Here's how the part is built. I have some questions about the finished solid (model axes, mm). Coordinates: 2 decimals unless noted, no trailing zeros. Loops run counter-clockwise (first coordinate to the right, second up) from the corner with the lowest first, then second, coordinate; pieces in that order, holes last. Notation, with made-up numbers: M 40.25,32 L 99.25,32 A32 cw 99.25,71 Z; hole C 43.25,60 d10. An arc over 180 degrees is marked long. Use one line per item in the form item = value. Start each with the question number.
(1) Imagine slicing it at D-D, the plane z = 3.35. Please give me the cut outline in (x, y), and give its area (3 significant figures).
(2) Imagine slicing it at C-C, the plane y = -6. Please give me the cut outline in (x, z), and give its area (3 significant figures).
(3) Please list where these lines run through material, in increasing order: L1, parallel to Y at x = 0, z = 3.55; L2, parallel to X at y = 6, z = 2.3; L3, parallel to Y at x = 11.5, z = 0.3.
(4) Will these pins go through, and if not, where does the flat tip stop? P1, Ø2.5, axis at x = 0, y = -12, coming from the +Z side; P2, Ø3, axis at y = 6, z = 2.5, coming from the -X side.
(5) Imagine slicing it at B-B, the plane y = 0. Please give me the cut outline in (x, z).
(6) Thinking about a two-plate mould opening in Y: for faces 1 (the flat face through (8, 0, 5)), 2 (the cylindrical face through (11.701, -4.294, 2.465)), 3 (the cylindrical face through (-4.01, 18.06, 2.46)), which applies, +Y half, -Y half, draft (parallel to the pull), parting line (faces both ways), or undercut?
(7) Imagine slicing it at A-A, the plane x = 0. Please give me the cut outline in (y, z), and give its area (3 significant figures).
Autodesk Inventor part; units mm, degrees
ref_plane "YZ Plane" through (0, 0, 0) normal (1, 0, 0) x (0, 1, 0)
ref_plane "XZ Plane" through (0, 0, 0) normal (0, 1, 0) x (-1, 0, 0)
ref_plane "XY Plane" through (0, 0, 0) normal (0, 0, 1) x (1, 0, 0)
sketch "スケッチ1" plane through (0, 0, 0) normal (0, 0, 1) x (1, 0, 0)
  circle A0 centre (0, 0) radius 18.5
  dimension "d0" = 37
extrude "押し出し1" add sketch "スケッチ1" along normal blind 5
sketch "スケッチ2" plane through (0, 0, 5) normal (0, 0, 1) x (1, 0, 0)
  circle A0 centre (0, 0) radius 12
  point P0 (0, 12)
  point P1 (-10.3923, 6)
  point P2 (-10.3923, -6)
  point P3 (0, -12)
  point P4 (10.3923, -6)
  point P5 (10.3923, 6)
  dimension "d3" = 24
  dimension "d6" = 360
hole "穴1" at (0, 12, 5) at (-10.3923, 6, 5) at (-10.3923, -6, 5) at (0, -12, 5) at (10.3923, -6, 5) at (10.3923, 6, 5) direction (0, 0, -1) diameter 4.3 end through all
sketch "スケッチ3" plane through (0, 0, 5) normal (0, 0, 1) x (1, 0, 0)
  circle A0 centre (0, 0) radius 7
  dimension "d15" = 14
extrude "押し出し2" cut sketch "スケッチ3" against normal blind 5
properties part number "servoplate_forR6" material "アルミニウム 6061"
Answer:
q1.outline = C 0,0 d37; hole C -10.39,-6 d4.3; hole C -10.39,6 d4.3; hole C 0,0 d14; hole C 0,-12 d4.3; hole C 0,12 d4.3; hole C 10.39,-6 d4.3; hole C 10.39,6 d4.3
q1.area = 834 mm²
q2.outline = M -17.5,0 L -12.54,0 L -12.54,5 L -17.5,5 Z; M -8.24,0 L -3.61,0 L -3.61,5 L -8.24,5 Z; M 3.61,0 L 8.24,0 L 8.24,5 L 3.61,5 Z; M 12.54,0 L 17.5,0 L 17.5,5 L 12.54,5 Z
q2.area = 95.9 mm²
q3.L1 = -18.5 to -14.15, -9.85 to -7, 7 to 9.85, 14.15 to 18.5
q3.L2 = -17.5 to -12.54, -8.24 to -3.61, 3.61 to 8.24, 12.54 to 17.5
q3.L3 = -14.49 to -7.84, -4.16 to 4.16, 7.84 to 14.49
q4.P1 = through
q4.P2 = -17.94
q5.outline = M -18.5,0 L -7,0 L -7,5 L -18.5,5 Z; M 7,0 L 18.5,0 L 18.5,5 L 7,5 Z
q6.face_1 = draft
q6.face_2 = undercut
q6.face_3 = parting line
q7.outline = M -18.5,0 L -14.15,0 L -14.15,5 L -18.5,5 Z; M -9.85,0 L -7,0 L -7,5 L -9.85,5 Z; M 7,0 L 9.85,0 L 9.85,5 L 7,5 Z; M 14.15,0 L 18.5,0 L 18.5,5 L 14.15,5 Z
q7.area = 72.0 mm²
